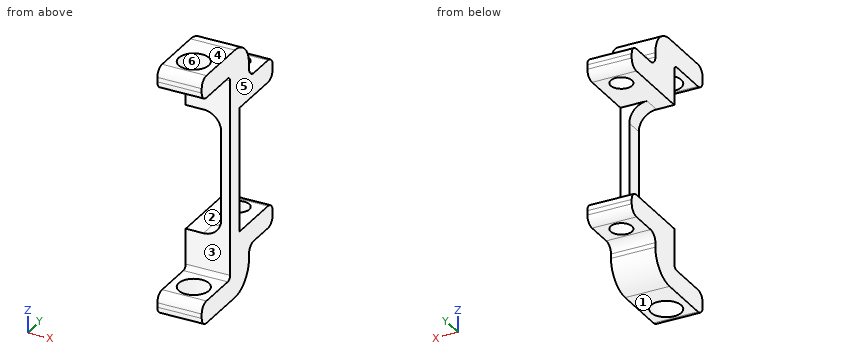
Autodesk Inventor part; units mm, degrees
ref_plane "YZ Plane" through (0, 0, 0) normal (1, 0, 0) x (0, 1, 0)
ref_plane "XZ Plane" through (0, 0, 0) normal (0, 1, 0) x (-1, 0, 0)
ref_plane "XY Plane" through (0, 0, 0) normal (0, 0, 1) x (1, 0, 0)
sketch "Эскиз1" plane through (0, 0, 0) normal (0, 1, 0) x (-1, 0, 0)
  line L0 (-7, -7) -> (7, -7)
  line L1 (7, -7) -> (7, 7)
  line L2 (7, 7) -> (-7, 7)
  line L3 (-7, 7) -> (-7, -7)
  line L4 (-7, -7) -> (7, 7) construction
  line L5 (7, -7) -> (-7, 7) construction
  line L6 (-14, -14) -> (14, -14)
  line L7 (14, -14) -> (14, 14)
  line L8 (14, 14) -> (-14, 14)
  line L9 (-14, 14) -> (-14, -14)
  line L10 (-14, -14) -> (14, 14) construction
  line L11 (14, -14) -> (-14, 14) construction
  point P0 (0, 0)
  dimension "d0" = 14
  dimension "d1" = 14
  dimension "d2" = 28
  dimension "d3" = 28
extrude "Выдавливание1" add sketch "Эскиз1" along normal blind 15
sketch "Эскиз2" plane through (0, 15, 0) normal (0, 1, 0) x (1, 0, 0)
  line L0 (9.5, 9.5) -> (-9.5, 9.5)
  line L1 (-9.5, 9.5) -> (-9.5, -9.5)
  line L2 (-9.5, -9.5) -> (9.5, -9.5)
  line L3 (9.5, -9.5) -> (9.5, 9.5)
  line L4 (9.5, 9.5) -> (-9.5, -9.5) construction
  line L5 (-9.5, 9.5) -> (9.5, -9.5) construction
  line L6 (-14, 14) -> (-14, -14)
  line L7 (14, 14) -> (-14, 14)
  line L8 (-14, 14) -> (-14, -14)
  line L9 (-14, -14) -> (14, -14)
  line L10 (14, -14) -> (14, 14)
  line L11 (14, 14) -> (-14, -14) construction
  line L12 (-14, 14) -> (14, -14) construction
  point P0 (0, 0)
  dimension "d6" = 19
  dimension "d7" = 19
extrude "Выдавливание2" cut sketch "Эскиз2" against normal blind 5
sketch "Эскиз4" plane through (-9.5, 15, 9.5) normal (0, 0, 1) x (1, 0, 0)
  point P0 (9.5, -15)
  point P1 (9.5, -2.5)
hole "Отверстие1" at (0, 12.5, 9.5) direction (0, 0, -1) diameter 2.4 end through all
sketch "Эскиз5" plane through (-14, 0, 14) normal (0, 0, 1) x (1, 0, 0)
  point P0 (14, 0)
  point P1 (14.0165, 2.9909)
hole "Отверстие2" at (0.0165, 2.9909, 14) direction (0, 0, -1) diameter 3.4 end through all
sketch "Эскиз6" plane through (0, 0, 0) normal (0, -1, 0) x (1, 0, 0)
  line L0 (11.5, -11.5) -> (-11.5, -11.5)
  line L1 (-11.5, -11.5) -> (-11.5, 11.5)
  line L2 (-11.5, 11.5) -> (11.5, 11.5)
  line L3 (11.5, 11.5) -> (11.5, -11.5)
  line L4 (11.5, -11.5) -> (-11.5, 11.5) construction
  line L5 (-11.5, -11.5) -> (11.5, 11.5) construction
  point P0 (0, 0)
  dimension "d24" = 23
  dimension "d25" = 23
extrude "Выдавливание3" cut sketch "Эскиз6" against normal blind 6
sketch "Эскиз7" plane through (-14, 0, -14) normal (-1, 0, 0) x (0, 0, 1)
  line L0 (28, 0) -> (28, 10)
  line L1 (28, 0) -> (0, 0)
  line L2 (0, 0) -> (0, 15.2302)
  line L3 (0, 15.2302) -> (28, 15.2302)
  line L4 (28, 15.2302) -> (28, 0)
  point P0 (14, 0)
extrude "Выдавливание4" cut sketch "Эскиз7" against normal blind 11.5
sketch "Эскиз8" plane through (14, 0, 14) normal (1, 0, 0) x (0, 0, -1)
  line L0 (0, 0) -> (28, 0)
  line L1 (28, 0) -> (0, 0)
  line L2 (0, 0) -> (0, 16.0654)
  line L3 (0, 16.0654) -> (28, 16.0654)
  line L4 (28, 16.0654) -> (28, 0)
  point P0 (14, 0)
extrude "Выдавливание5" cut sketch "Эскиз8" against normal blind 11.5
sketch "Эскиз9" plane through (-2.5, 6, 7) normal (0, 0, -1) x (-1, 0, 0)
  line L0 (-5, 9) -> (-5, 0)
  line L1 (-5, 0) -> (-4, 0)
  line L2 (-4, 0) -> (-4, 2)
  line L3 (-4, 2) -> (-5, 2)
  line L4 (-5, 2) -> (-5, 0)
  point P0 (-2.5, -6)
  dimension "d32" = 1
  dimension "d35" = 2
extrude "Выдавливание6" add sketch "Эскиз9" along normal blind 14
fillet "Сопряжение1" radius 2 2 edges at (1.5, 7, 7) (1.5, 7, -7)
fillet "Сопряжение1" radius 1 10 edges at (0, 15, 9.5) (0, 15, 7) (0, 15, -9.5) (0, 15, -7) (0, 10, -9.5) (0, 10, 9.5) (0, 0, 11.5) (0, 0, 14) (0, 0, -14) (0, 0, -11.5)
fillet "Сопряжение1" radius 0.5 2 edges at (0, 6, 11.5) (0, 6, -11.5)
fillet "Сопряжение1" radius 3 2 edges at (0, 10, -14) (0, 10, 14)
properties part number "14mmto28mm"
Work out the finished part from the listing and answer in its coordinate system (mm). Face numbers are marked on the shaded views. A direction names the side the tool comes from. Give positions to 0.01 mm unless a question says otherwise; leave off trailing zeros. Order: outer loops, then holes, each group sorted by start corner. A loop starts at its lowest first (then second) coordinate and runs counter-clockwise, first axis right, second up. Notation, with made-up numbers: (36, -0.75) - (88, -0.75) arc R24 cw to (88, 12.25) - close; hole circle Ø1 at (-34.75, 4.5). An arc over 180 degrees is marked (long way). Answer as CSV lines item,"result". Start each with the question number.
Q1. The part is cut by section C-C (z = -12). Write down the section's boundary in (x, y).
Q2. Find the intervals of material crossed by L1, parallel to X at y = 12.5, z = 7.6; L2, parallel to Z at x = -1, y = 6.25; L3, parallel to Y at x = 0, z = -8.35, in increasing order. Write a range as [from, to].
Q3. The mould has two halves that part along X. Classify the marked faces 4, 5 and 6: +X half, -X half, draft (parallel to the pull), parting line (faces both ways), or undercut.
Q4. The part is cut by section A-A (y = 2). Write down the section's boundary in (x, z).
Q5. The part is cut by section D-D (y = 12.5). Write down the section's boundary in (x, z), then the cut area to 3 significant figures.
Q6. For the marked faces 1, 2 and 3, determine the directions among +Z, -Z, +X, -X, +Y, -Y from which every point of the face is accessible in a straight line to the end or side of a thin tool.
Q7. The part is cut by section B-B (y = 10.5). Write down the section's boundary in (x, z).
Q8. Given pin 1 Ø1 at (y, z) = (6.5, 2) entering from -X; pin 2 Ø3 at (x, y) = (0, 12.5) entering from -Z; pin 3 Ø0.6 at (x, z) = (-0.5, -10.5) entering from +Y, each flat-ended and moving along its own axis, determine where each tip first touches the part or whether it passes through.
Check result:
1,outline,"(-2.5, 0.13) - (2.5, 0.13) - (2.5, 9.83) - (-2.5, 9.83) - close; hole circle Ø3.4 at (0.02, 2.99)"
2,L1,"x = [-2.5, -1.2], [1.2, 2.5]"
2,L2,"z = [-14, -7], [7, 14]"
2,L3,"y = [6, 11.3], [13.7, 15]"
3,face 4,"draft"
3,face 5,"+X half"
3,face 6,"undercut"
4,outline,"(-2.5, -14) - (-1.36, -14) - (-1.36, -11.5) - (-2.5, -11.5) - close; (-2.5, 11.5) - (-1.36, 11.5) - (-1.36, 14) - (-2.5, 14) - close; (1.4, -14) - (2.5, -14) - (2.5, -11.5) - (1.4, -11.5) - close; (1.4, 11.5) - (2.5, 11.5) - (2.5, 14) - (1.4, 14) - close"
5,outline,"(-2.5, -9.5) - (-1.2, -9.5) - (-1.2, -7) - (-2.5, -7) - close; (-2.5, 7) - (-1.2, 7) - (-1.2, 9.5) - (-2.5, 9.5) - close; (1.2, -9.5) - (2.5, -9.5) - (2.5, -7) - (1.2, -7) - close; (1.2, 7) - (2.5, 7) - (2.5, 9.5) - (1.2, 9.5) - close"
5,area,"13.0 mm²"
6,face 1,"-Z, +X, -X, +Y, -Y"
6,face 2,"-X, +Y"
6,face 3,"+X, -X, -Y"
7,outline,"(-2.5, -9.63) - (2.5, -9.63) - (2.5, -7) - (-2.5, -7) - close; (-2.5, 7) - (2.5, 7) - (2.5, 9.63) - (-2.5, 9.63) - close"
8,pin 1,"stops at x = 1.5"
8,pin 2,"stops at z = -9.5"
8,pin 3,"stops at y = 10.05"
